from build123d import *

# Parameters (mm, degrees)
F0_W     = 13.5
F0_H     = 1.8
F0_H_2   = 15.4
F0_W_2   = 8.2
F0_H_3   = 13.6
F1_DEPTH = 2.4
F2_DEPTH = 141.6
F3_R     = 8
F4_R     = 9.6
F5_R     = 2
F6_R     = 1


with BuildPart() as f1:
    # F0 (on Top) → F1 (new body)
    with BuildSketch(Plane.XY):
        Polygon((-13.5, -1.8), (-13.5, 0), (-15.3, 0), (-15.3, -17.2), (-13.5, -17.2), align=None)
        with Locations((-6.75, -0.9)):
            Rectangle(F0_W, F0_H)
        with Locations((-6.75, -9.5)):
            Rectangle(F0_W, F0_H_2)
        Polygon((1.8, -1.8), (0, -1.8), (0, -17.2), (1.8, -17.2), (1.8, -15.4), align=None)
        with Locations((5.9, -16.3)):
            Rectangle(F0_W_2, F0_H)
        with Locations((5.9, -8.6)):
            Rectangle(F0_W_2, F0_H_3)
        Polygon((10, 0), (0, 0), (0, -1.8), (1.8, -1.8), (10, -1.8), align=None)
    extrude(amount=-F1_DEPTH)

    # F0 (on Top) → F2 (join)
    with BuildSketch(Plane.XY):
        Polygon((-13.5, -1.8), (-13.5, 0), (-15.3, 0), (-15.3, -17.2), (-13.5, -17.2), align=None)
        Polygon((1.8, -1.8), (0, -1.8), (0, -17.2), (1.8, -17.2), (1.8, -15.4), align=None)
        with Locations((-6.75, -0.9)):
            Rectangle(F0_W, F0_H)
        Polygon((10, 0), (0, 0), (0, -1.8), (1.8, -1.8), (10, -1.8), align=None)
        with Locations((5.9, -16.3)):
            Rectangle(F0_W_2, F0_H)
    extrude(amount=F2_DEPTH)

    # F3
    f3_edges = [f1.edges().sort_by_distance(p)[0] for p in [
        (-13.5, -1.8, 70.8),
    ]]
    fillet(f3_edges, radius=F3_R)

    # F4
    f4_edges = [f1.edges().sort_by_distance(p)[0] for p in [
        (-15.3, 0, 69.6),
    ]]
    fillet(f4_edges, radius=F4_R)

    # F5
    f5_edges = [f1.edges().sort_by_distance(p)[0] for p in [
        (0, -1.8, 70.8),
        (1.8, -1.8, 70.8),
        (1.8, -15.4, 70.8),
    ]]
    fillet(f5_edges, radius=F5_R)

    # F6
    f6_edges = [f1.edges().sort_by_distance(p)[0] for p in [
        (6.9, -15.4, 0),
        (2.385786, -14.814214, 0),
        (1.8, -8.6, 0),
        (2.385786, -2.385786, 0),
        (6.9, -1.8, 0),
        (0, -10.5, 0),
        (-0.585786, -2.385786, 0),
        (-3.75, -1.8, 0),
        (-11.156854, -4.143146, 0),
        (-13.5, -13.5, 0),
    ]]
    fillet(f6_edges, radius=F6_R)


solid = f1.part
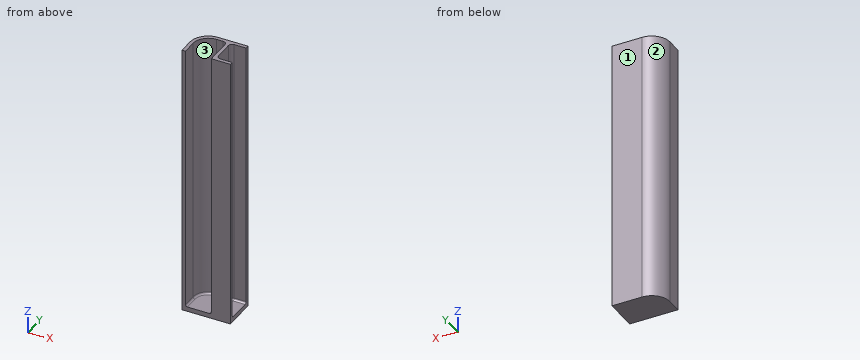
Here's how the part is built. I have some questions about the finished solid (model axes, mm). Face numbers are marked on the shaded views. Coordinates: 2 decimals unless noted, no trailing zeros. Order: outer loops, then holes, each group sorted by start corner. A loop starts at its lowest first (then second) coordinate and runs counter-clockwise, first axis right, second up. Notation, with made-up numbers: M 26,73 L 43,73 A22 cw 43,81 Z; hole C 4.25,-6.5 d9. An arc over 180 degrees is marked long. Answer as CSV lines item,"result". Start each with the question number.
1. We'd pull the mould along X, two halves only. Please class the marked faces 1, 2 and 3: released by +X, released by -X, zero draft, split by the parting line, or undercut.
2. I want a section at B-B, the plane x = -3.75. Write out the boundary of the cut face in (y, z).
3. I want a section at A-A, the plane z = 29.5. Write out the boundary of the cut face in (x, y).
4. I need wall thicknesses on line 1 (X direction, y = -9.25, z = 30); line 2 (Y direction, x = 7.25, z = 69.5); line 3 (Y direction, x = -2.75, z = 86). Which ranges of each line are inside material? Lowest first, please. Write a range as [from, to].
5. For pin 1 (7.5 mm diameter, centred on y = -10.5, z = 36.5, fed in from +X); pin 2 (4 mm diameter, centred on x = -4, z = 65.5, fed in from -Y); pin 3 (5 mm diameter, centred on x = -9, y = -10.5, fed in from +Z), each with a flat end and sliding along its axis, tell me the tip position at first contact or that it passes through.
Recorded:
1,face 1,"zero draft"
1,face 2,"released by -X"
1,face 3,"undercut"
2,outline,"M -17.2,-2.4 L 0,-2.4 L 0,141.6 L -1.8,141.6 L -1.8,1 A1 cw -2.8,0 L -17.2,0 Z"
3,outline,"M -15.3,-17.2 L -13.5,-17.2 L -13.5,-9.8 A8 cw -5.5,-1.8 L -2,-1.8 A2 cw 0,-3.8 L 0,-17.2 L 10,-17.2 L 10,-15.4 L 3.8,-15.4 A2 cw 1.8,-13.4 L 1.8,-3.8 A2 cw 3.8,-1.8 L 10,-1.8 L 10,0 L -5.7,0 A9.6 ccw -15.3,-9.6 Z"
4,line 1,"x = [-15.29, -13.48], [0, 1.8]"
4,line 2,"y = [-17.2, -15.4], [-1.8, 0]"
4,line 3,"y = [-1.8, 0]"
5,pin 1,"stops at x = 1.99"
5,pin 2,"stops at y = -1.82"
5,pin 3,"stops at z = 0"
